```python
from build123d import *

# Parameters (mm, degrees)
SKETCH1_W           = 50
SKETCH1_H           = 52
SKETCH1_R           = 11
SKETCH1_R_2         = 1.5
BOSS_EXTRUDE1_DEPTH = 3
CHAMFER1_SIZE       = 4
SKETCH2_W           = 50
SKETCH2_H           = 3
BOSS_EXTRUDE2_DEPTH = 50
BOSS_EXTRUDE3_DEPTH = 2
BOSS_EXTRUDE4_DEPTH = 2
CHAMFER2_SIZE       = 4
CUT_EXTRUDE1_DEPTH  = 4


with BuildPart() as part:
    # Sketch1 → Boss-Extrude1 (new body)
    with BuildSketch(Plane.XY):
        Rectangle(SKETCH1_W, SKETCH1_H)
        with Locations((0, 5)):
            Circle(SKETCH1_R, mode=Mode.SUBTRACT)
        with Locations((-15.5, 20.5)):
            Circle(SKETCH1_R_2, mode=Mode.SUBTRACT)
        with Locations((15.5, 20.5)):
            Circle(SKETCH1_R_2, mode=Mode.SUBTRACT)
        with Locations((15.5, -10.5)):
            Circle(SKETCH1_R_2, mode=Mode.SUBTRACT)
        with Locations((-15.5, -10.5)):
            Circle(SKETCH1_R_2, mode=Mode.SUBTRACT)
    extrude(amount=BOSS_EXTRUDE1_DEPTH)

    # Chamfer1
    chamfer1_edges = [part.edges().sort_by_distance(p)[0] for p in [
        (-25, 26, 1.5),
        (25, 26, 1.5),
    ]]
    chamfer(chamfer1_edges, length=CHAMFER1_SIZE)

    # Sketch2 → Boss-Extrude2 (add)
    with BuildSketch(Plane.XY.offset(3)):
        with Locations((0, -24.5)):
            Rectangle(SKETCH2_W, SKETCH2_H)
    extrude(amount=BOSS_EXTRUDE2_DEPTH)

    # Sketch3 → Boss-Extrude3 (add)
    with BuildSketch(Plane(origin=(25, 0, 0), x_dir=(0, 0, -1), z_dir=(1, 0, 0))):
        Polygon((-3, -13), (-11, -23), (-3, -23), align=None)
    extrude(amount=-BOSS_EXTRUDE3_DEPTH)

    # Sketch4 → Boss-Extrude4 (add)
    with BuildSketch(Plane.ZY.offset(25)):
        Polygon((3, -13), (3, -23), (11, -23), align=None)
    extrude(amount=-BOSS_EXTRUDE4_DEPTH)

    # Chamfer2
    chamfer2_edges = [part.edges().sort_by_distance(p)[0] for p in [
        (-25, -24.5, 53),
        (25, -24.5, 53),
    ]]
    chamfer(chamfer2_edges, length=CHAMFER2_SIZE)

    # Sketch5 → Cut-Extrude1 (cut, through all)
    with BuildSketch(Plane(origin=(0, -23, 0), x_dir=(1, 0, 0), z_dir=(0, 1, 0))):
        with BuildLine():
            Line((-13, -15), (-13, -45))
            ThreePointArc((-13, -45), (-15, -47), (-17, -45))
            Line((-17, -45), (-17, -15))
            ThreePointArc((-17, -15), (-15, -13), (-13, -15))
        make_face()
        with BuildLine():
            Line((13, -15), (13, -45))
            ThreePointArc((13, -45), (15, -47), (17, -45))
            Line((17, -45), (17, -15))
            ThreePointArc((17, -15), (15, -13), (13, -15))
        make_face()
    extrude(amount=-CUT_EXTRUDE1_DEPTH, mode=Mode.SUBTRACT)


solid = part.part
```
Model file for the job. Use its own axes, mm. A direction names the side the tool comes from. Coordinates: 2 decimals unless noted, no trailing zeros. Loops run counter-clockwise (first coordinate to the right, second up) from the corner with the lowest first, then second, coordinate; pieces in that order, holes last. Notation, with made-up numbers: (-23, 37.5) -> (36, 37.5) arc R33 cw to (36, 74.5) -> close; hole circle Ø3 at (75.25, 73). An arc over 180 degrees is marked (long way). Answer as a JSON object with one key per item and string values.
Q1. Pull direction Y, two halves, no side cores. Call faces 4 (the cylindrical face through (-16.61, 21.51, 1.48)), 5 (the flat face through (-24, -18, 7)), 6 (the flat face through (-13, -24, 30)), 7 (the cylindrical face through (14.3, -11.4, 1.5)): released by +Y, released by -Y, zero draft, split by the parting line, or undercut.
Report:
{"face 4": "undercut", "face 5": "released by +Y", "face 6": "zero draft", "face 7": "undercut"}
Q2. Cut at C-C (x = -15.5). List the corners of the cut face in (y, z), and give its area (3 significant figures).
Report:
{"outline": "(-26, 0) -> (-12, 0) -> (-12, 3) -> (-23, 3) -> (-23, 13.06) -> (-26, 13.06) -> close; (-26, 46.94) -> (-23, 46.94) -> (-23, 53) -> (-26, 53) -> close; (-9, 0) -> (19, 0) -> (19, 3) -> (-9, 3) -> close; (22, 0) -> (26, 0) -> (26, 3) -> (22, 3) -> close", "area": "186 mm2"}
Q3. Cut at B-B (z = 42). List the corners of the cut face in (x, y).
Report:
{"outline": "(-25, -26) -> (-17, -26) -> (-17, -23) -> (-25, -23) -> close; (-13, -26) -> (13, -26) -> (13, -23) -> (-13, -23) -> close; (17, -26) -> (25, -26) -> (25, -23) -> (17, -23) -> close"}
Q4. Flat gauge pins, fed straight in: P1, Ø6, axis at x = -7, y = -19, coming from the +Z side; P2, Ø1.5, axis at x = 5.5, z = 30.5, coming from the +Y side. Where does each tip first touch, or does it go through?
Report:
{"P1": "stops at z = 3", "P2": "stops at y = -23"}
Q5. Cut at A-A (y = 5). List the corners of the cut face in (x, z), and give its area (3 significant figures).
Report:
{"outline": "(-25, 0) -> (-11, 0) -> (-11, 3) -> (-25, 3) -> close; (11, 0) -> (25, 0) -> (25, 3) -> (11, 3) -> close", "area": "84.0 mm2"}
Q6. Cut at D-D (y = 20.5). List the corners of the cut face in (x, z).
Report:
{"outline": "(-25, 0) -> (-17, 0) -> (-17, 3) -> (-25, 3) -> close; (-14, 0) -> (14, 0) -> (14, 3) -> (-14, 3) -> close; (17, 0) -> (25, 0) -> (25, 3) -> (17, 3) -> close"}
Q7. 3-axis set-ups, long thin cutter, end or side, ignore diameter. For faces 1 (the cylindrical face through (15, -24, 13)), 2 (the flat face through (-23, 24, 1)), 3 (the flat face through (0, -23, 28)): which of +Z, -Z, +X, -X, +Y, -Y reach the whole face in a straight line?
Report:
{"face 1": "+Y, -Y", "face 2": "+Z, -Z, -X, +Y", "face 3": "+Z, +Y"}
Q8. Probe probe 1 along Y at (x, z) = (-15.5, 2.05); probe 2 along X at (y, z) = (-20, 5.5); probe 3 along Z at (x, y) = (6, 23). List the from-to ranges inside material, lowest first.
Report:
{"probe 1": "y = -26 to -12, -9 to 19, 22 to 26", "probe 2": "x = -25 to -23, 23 to 25", "probe 3": "z = 0 to 3"}
